Verification items for the finished model (mm, model axes). Face numbers are marked on the shaded views. Coordinates: 2 decimals unless noted, no trailing zeros. Order: outer loops, then holes, each group sorted by start corner. A loop starts at its lowest first (then second) coordinate and runs counter-clockwise, first axis right, second up. Notation, with made-up numbers: M 73,75.5 L 127,75.5 A21 ccw 127,110.5 Z; hole C 4.25,78.5 d1. An arc over 180 degrees is marked long. Answer as a JSON object with one key per item and string values. Group by question number.
(1) Cross-section at D-D (x = -3). Enter the section's corners in (y, z).
(2) Cross-section at C-C (y = -10). Enter the section's corners in (x, z) (3 decimals), plus the area to 3 significant figures.
(3) Gauge pin test, flat ends, axial feed: pin 1 Ø8 at (x, y) = (5.5, -21) entering from +Z; pin 2 Ø8 at (x, y) = (10, -16) entering from +Z; pin 3 Ø15 at (x, y) = (11, -15) entering from -Z; pin 4 Ø1.1 at (y, z) = (-15, 66) entering from -X. Record the tip position at first contact, or that the pin passes through.
(4) Mould release check, pull along Y, two halves, no side actions. Record for the marked faces 1, 2, 3 and 4: released by +Y, released by -Y, zero draft, split by the parting line, or undercut.
(5) Cross-section at B-B (z = 22.5). Enter the section's corners in (x, y).
(6) Material ranges on line 1 (Y direction, x = 11, z = 1.75); line 2 (Z direction, x = -18.5, y = -14.75); line 3 (Y direction, x = 11, z = -8), recorded low to high.
(7) Cross-section at A-A (x = 11). Enter the section's corners in (y, z), plus the area to 3 significant figures.
from build123d import *

# Parameters (mm, degrees)
F0_W     = 70
F0_H     = 23.5
F1_DEPTH = 30
F2_R     = 8
F3_DEPTH = 19.5
F4_R     = 7.5
F5_DEPTH = 2
F6_R     = 6.5
F7_DEPTH = 2.001
F8_W     = 5
F8_H     = 5
F9_DEPTH = 85
F10_R    = 2


with BuildPart() as f1:
    # F0 (on Front) → F1 (new body)
    with BuildSketch(Plane.XZ):
        Rectangle(F0_W, F0_H)
    extrude(amount=F1_DEPTH)

    # F2 (on face) → F3 (cut)
    with BuildSketch(Plane.XY.offset(11.75)):
        with Locations((11, -15)):
            Circle(F2_R)
    extrude(amount=-F3_DEPTH, mode=Mode.SUBTRACT)

    # F4 (on face) → F5 (cut)
    with BuildSketch(Plane.XY.offset(-7.75)):
        with Locations((11, -15)):
            Circle(F4_R)
    extrude(amount=-F5_DEPTH, mode=Mode.SUBTRACT)

    # F6 (on face) → F7 (cut, through all)
    with BuildSketch(Plane.XY.offset(-9.75)):
        with Locations((11, -15)):
            Circle(F6_R)
    extrude(amount=-F7_DEPTH, mode=Mode.SUBTRACT)

    # F8 (on face) → F9 (join)
    with BuildSketch(Plane.XY.offset(11.75)):
        with Locations((-30, -15)):
            Rectangle(F8_W, F8_H)
    extrude(amount=F9_DEPTH)

    # F10
    f10_edges = [f1.edges().sort_by_distance(p)[0] for p in [
        (0, -30, 11.75),
        (35, -15, 11.75),
        (35, -30, 0),
        (35, 0, 0),
        (35, -15, -11.75),
        (0, 0, 11.75),
        (0, 0, -11.75),
        (-35, 0, 0),
        (-35, -15, 11.75),
        (-35, -30, 0),
        (-35, -15, -11.75),
        (0, -30, -11.75),
        (-32.5, -17.5, 54.25),
        (-27.5, -17.5, 54.25),
        (-27.5, -12.5, 54.25),
        (-32.5, -12.5, 54.25),
    ]]
    fillet(f10_edges, radius=F10_R)


solid = f1.part
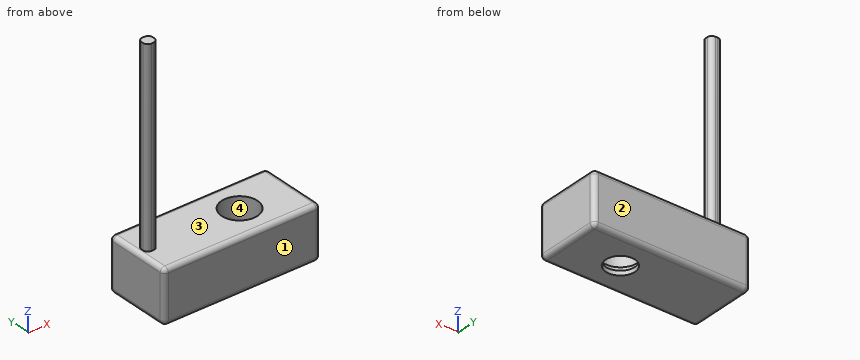
Taken from the geometry:
{
 "1": {"outline": "M -30,-9.75 A2 ccw -28,-11.75 L -2,-11.75 A2 ccw 0,-9.75 L 0,9.75 A2 ccw -2,11.75 L -28,11.75 A2 ccw -30,9.75 Z"},
 "2": {"outline": "M -35,-9.75 A2 ccw -33,-11.75 L 6.847,-11.75 L 6.847,-9.75 L 5.41,-9.75 L 5.41,-7.75 L 4.755,-7.75 L 4.755,11.75 L -33,11.75 A2 ccw -35,9.75 Z; M 15.153,-11.75 L 33,-11.75 A2 ccw 35,-9.75 L 35,9.75 A2 ccw 33,11.75 L 17.245,11.75 L 17.245,-7.75 L 16.59,-7.75 L 16.59,-9.75 L 15.153,-9.75 Z", "area": "1,360 mm²"},
 "3": {"pin 1": "stops at z = 11.75", "pin 2": "passes through", "pin 3": "stops at z = -11.75", "pin 4": "stops at x = -32.5"},
 "4": {"face 1": "released by -Y", "face 2": "released by +Y", "face 3": "zero draft", "face 4": "undercut"},
 "5": {"outline": "M -32.5,-15.5 A2 ccw -30.5,-17.5 L -29.5,-17.5 A2 ccw -27.5,-15.5 L -27.5,-14.5 A2 ccw -29.5,-12.5 L -30.5,-12.5 A2 ccw -32.5,-14.5 Z"},
 "6": {"line 1": "y = -30 to -23, -7 to 0", "line 2": "z = -11.75 to 11.75", "line 3": "y = -30 to -22.5, -7.5 to 0"},
 "7": {"outline": "M -30,-9.75 A2 ccw -28,-11.75 L -21.5,-11.75 L -21.5,-9.75 L -22.5,-9.75 L -22.5,-7.75 L -23,-7.75 L -23,11.75 L -28,11.75 A2 ccw -30,9.75 Z; M -8.5,-11.75 L -2,-11.75 A2 ccw 0,-9.75 L 0,9.75 A2 ccw -2,11.75 L -7,11.75 L -7,-7.75 L -7.5,-7.75 L -7.5,-9.75 L -8.5,-9.75 Z", "area": "334 mm²"}
}
